Could you check a few things on this model? Use its own coordinates, in mm. A direction names the side the tool comes from. Give positions to 0.01 mm unless a question says otherwise; leave off trailing zeros. Write each loop counter-clockwise with the first axis right and the second up, starting at its lowest first coordinate (ties: lowest second). Pieces come first, ordered by that corner, then holes. Notation, with made-up numbers: (18.5, -25.5) -> (66.5, -25.5) arc R25 cw to (66.5, 7.5) -> close; hole circle Ø11 at (30, 16.25). An arc over 180 degrees is marked (long way). Write item = value, one per line. Start each with the question number.
Solid Edge part; units mm, degrees
sketch "Sketch1" plane through (0, 0, 0) normal (0, -1, 0) x (1, 0, 0)
  line L0 (0, 0) -> (-21.8382, 60)
  line L1 (-21.8382, 60) -> (-21.8382, 70)
  line L2 (-21.8382, 70) -> (-38.1618, 70)
  line L3 (-38.1618, 60) -> (-38.1618, 70)
  line L4 (-60, 0) -> (-38.1618, 60)
  line L5 (0, 0) -> (-60, 0)
extrude "Protrusion1" add sketch "Sketch1" against normal blind 30
sketch "Sketch2" plane through (-21.8382, 15, 65) normal (1, 0, 0) x (0, 0, 1)
  line L0 (-5, 3) -> (5, 3)
  line L1 (5, 3) -> (5, -15)
  line L2 (5, -15) -> (-5, -15)
  line L3 (-5, -15) -> (-5, 3)
extrude "ExtrudedCutout_2" cut sketch "Sketch2" against normal blind 20
sketch "Sketch3" plane through (-10.9191, 15, 30) normal (0.9397, 0, 0.342) x (0, 1, 0)
  line L0 (-3, 31.9253) -> (15, -31.9253)
  line L1 (15, -31.9253) -> (15, 31.9253)
  line L2 (15, 31.9253) -> (-3, 31.9253)
extrude "ExtrudedCutout_3" cut sketch "Sketch3" against normal blind 68.6414
(1) We'd pull the mould along Z, two halves only. Please class faces 1 (the flat face through (-33, 30, 57)), 2 (the flat face through (-8.34, 11.46, 22.91)), 3 (the flat face through (-31.115, 21.126, 56.624)), 4 (the flat face through (-31.305, 20.874, 23.056)): released by +Z, released by -Z, zero draft, split by the parting line, or undercut.
(2) If I drill on line 1 along X through (y, z) = (2.25, 62); line 2 along X through (y, z) = (9.25, 56); line 3 along Y through (x, z) = (-15.5, 32.5), over which ranges is the centre line in solid material (lowest first)? Write a range as from..to.
(3) Imagine slicing it at B-B (x = -25). Please give me the cut outline in (y, z), then the cut area to 3 significant figures.
(4) Imagine slicing it at D-D (z = 55). Please give me the cut outline in (x, y).
(5) On a 3-axis mill with a long thin cutter (end or side, diameter ignored), from which of +Z, -Z, +X, -X, +Y, -Y can I reach the whole of each face in a straight line? I mean faces 5 (the flat face through (-30, 0, 28)), 6 (the flat face through (-30, 15, 0)), 7 (the flat face through (-30, 12, 65)), 8 (the flat face through (-21.838, 6, 65)), 9 (the flat face through (-38.162, 6, 65)). Say none if no direction works.
(6) I'm going to push flat-ended pins straight in: pin 1 (6 mm diameter, centred on y = 12, z = 61.5, fed in from +X); pin 2 (13 mm diameter, centred on x = -30.5, y = 21, fed in from +Z); pin 3 (4 mm diameter, centred on x = -45.5, z = 15.5, fed in from +Y). Where does each tip first touch, or does it pass through?
Answers below:
q1.face_1 = zero draft
q1.face_2 = released by +Z
q1.face_3 = undercut
q1.face_4 = undercut
q2.line_1 = -38.16..-21.84
q2.line_2 = -39.62..-20.38
q2.line_3 = 0..19.9
q3.outline = (0, 0) -> (27.59, 0) -> (12, 58.85) -> (30, 58.85) -> (30, 60) -> (12, 60) -> (12, 70) -> (0, 70) -> close
q3.area = 1,320 mm^2
q4.outline = (-39.98, 0) -> (-20.02, 0) -> (-20.02, 13.5) -> (-35.58, 12) -> (-35.58, 30) -> (-39.98, 30) -> close
q5.face_5 = +Z, -Z, +X, -X, -Y
q5.face_6 = -Z, +X, -X, +Y, -Y
q5.face_7 = +Z, +X, -X, +Y
q5.face_8 = +Z, +X, +Y, -Y
q5.face_9 = +Z, -X, +Y, -Y
q6.pin_1 = -21.29
q6.pin_2 = 60
q6.pin_3 = 22.07
